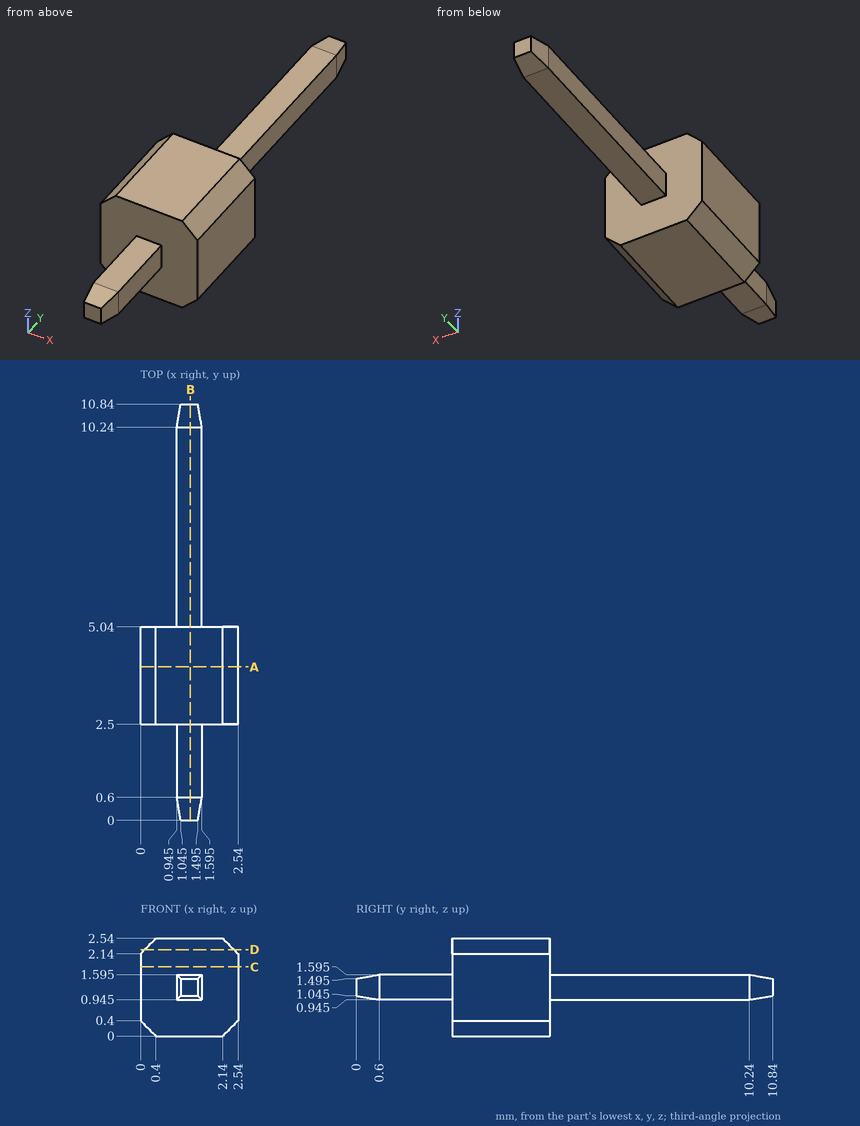
Check sheet for the drawn part. Datum: minimum x, y, z corner. Units: mm. Coordinates: 2 decimals unless noted, no trailing zeros. Loops run counter-clockwise (first coordinate to the right, second up) from the corner with the lowest first, then second, coordinate; pieces in that order, holes last. Notation, with made-up numbers: (41.25, 88) -> (87.25, 88) arc R21 ccw to (87.25, 114) -> close; hole circle Ø2 at (-40, 13). An arc over 180 degrees is marked (long way). Answer in a Markdown table with one row per item.
1. Sectioned sample at D-D, the plane z = 2.25. Record the boundary of the cut face in (x, y).
Check values:
| item | result |
|---|---|
| outline | (0.11, 2.5) -> (2.43, 2.5) -> (2.43, 5.04) -> (0.11, 5.04) -> close |
2. Sectioned sample at B-B, the plane x = 1.3. Record the boundary of the cut face in (y, z) (3 decimals).
Check values:
| item | result |
|---|---|
| outline | (0, 1.045) -> (0.6, 0.945) -> (2.5, 0.945) -> (2.5, 0) -> (5.04, 0) -> (5.04, 0.945) -> (10.24, 0.945) -> (10.84, 1.045) -> (10.84, 1.495) -> (10.24, 1.595) -> (5.04, 1.595) -> (5.04, 2.54) -> (2.5, 2.54) -> (2.5, 1.595) -> (0.6, 1.595) -> (0, 1.495) -> close |
3. Sectioned sample at C-C, the plane z = 1.8. Record the boundary of the cut face in (x, y).
Check values:
| item | result |
|---|---|
| outline | (0, 2.5) -> (2.54, 2.5) -> (2.54, 5.04) -> (0, 5.04) -> close |
4. Material ranges on line 1 along Y through (x, z) = (2.1, 0.6); line 2 along X through (y, z) = (2, 1.2) (3 decimals), recorded low to high. Write a range as [from, to].
Check values:
| item | result |
|---|---|
| line 1 | y = [2.5, 5.04] |
| line 2 | x = [0.945, 1.595] |
5. Sectioned sample at A-A, the plane y = 4. Record the boundary of the cut face in (x, z).
Check values:
| item | result |
|---|---|
| outline | (0, 0.4) -> (0.4, 0) -> (2.14, 0) -> (2.54, 0.4) -> (2.54, 2.14) -> (2.14, 2.54) -> (0.4, 2.54) -> (0, 2.14) -> close |
6. Go/stop test with flat-tipped pins: pin 1 (0.7 mm diameter, centred on x = 1, y = 1.5, fed in from +Z) (3 decimals); pin 2 (1.5 mm diameter, centred on y = 6.5, z = 0.5, fed in from +X) (3 decimals); pin 3 (0.7 mm diameter, centred on x = 1, y = 8.5, fed in from -Z) (3 decimals). Record where each tip stops, or that it passes through.
Check values:
| item | result |
|---|---|
| pin 1 | stops at z = 1.595 |
| pin 2 | stops at x = 1.595 |
| pin 3 | stops at z = 0.945 |
